```python
from build123d import *

# Parameters (mm, degrees)
SKETCH1_R                    = 4
BASE_FLANGE1_DEPTH           = 1.6002
EDGE_FLANGE1_STRIP_W         = 8.40080108
EDGE_FLANGE1_STRIP_H         = 1.6002
EDGE_FLANGE1_STRIP_CUT_DEPTH = 14
EDGE_FLANGE1_DEPTH           = 14
EDGE_FLANGE1_START           = 1.6002
EDGE_FLANGE1_PROFILE_R       = 2.5
EDGE_FLANGE1_FLAT_DEPTH      = 1.6002


# Sheet-metal steps are written as plain solids
with BuildPart() as part:
    # Sketch1 → Base-Flange1 (new body)
    with BuildSketch(Plane.XY):
        with BuildLine():
            Line((-7, -20), (-7, 0))
            ThreePointArc((-7, 0), (0, 7), (7, 0))
            Line((7, 0), (7, -20))
            Line((7, -20), (-7, -20))
        make_face()
        Circle(SKETCH1_R, mode=Mode.SUBTRACT)
    extrude(amount=-BASE_FLANGE1_DEPTH)

    # Edge-Flange1 strip (across the edge) → Edge-Flange1 strip cut (cut)
    with BuildSketch(Plane(origin=(-7, -20, 0), x_dir=(0, 1, 0), z_dir=(1, 0, 0))):
        with Locations((-3.2004, -0.8001)):
            Rectangle(EDGE_FLANGE1_STRIP_W, EDGE_FLANGE1_STRIP_H)
    extrude(amount=EDGE_FLANGE1_STRIP_CUT_DEPTH, mode=Mode.SUBTRACT)

    # Edge-Flange1 bend section (across the edge) → Edge-Flange1 (add)
    with BuildSketch(Plane(origin=(-7, -20, 0), x_dir=(0, 1, 0), z_dir=(1, 0, 0))):
        with BuildLine():
            Line((-1.6002, 1.00000054), (0, 1.00000054))
            ThreePointArc((0, 1.00000054), (0.292893377, 0.292893377), (1.00000054, 0))
            Line((1.00000054, 0), (1.00000054, -1.6002))
            ThreePointArc((1.00000054, -1.6002), (-0.838618894, -0.838618894), (-1.6002, 1.00000054))
        make_face()
    extrude(amount=EDGE_FLANGE1_DEPTH)

    # Edge-Flange1 profile (on flange) → Edge-Flange1 flat (add)
    with BuildSketch(Plane.XZ.offset(20).offset(EDGE_FLANGE1_START)):
        with BuildLine():
            ThreePointArc((7, 7), (0, 14), (-7, 7))
            Line((-7, 7), (-7, 1.00000054))
            Line((-7, 1.00000054), (7, 1.00000054))
            Line((7, 1.00000054), (7, 7))
        make_face()
        with Locations((0, 7)):
            Circle(EDGE_FLANGE1_PROFILE_R, mode=Mode.SUBTRACT)
    extrude(amount=-EDGE_FLANGE1_FLAT_DEPTH)


solid = part.part
```
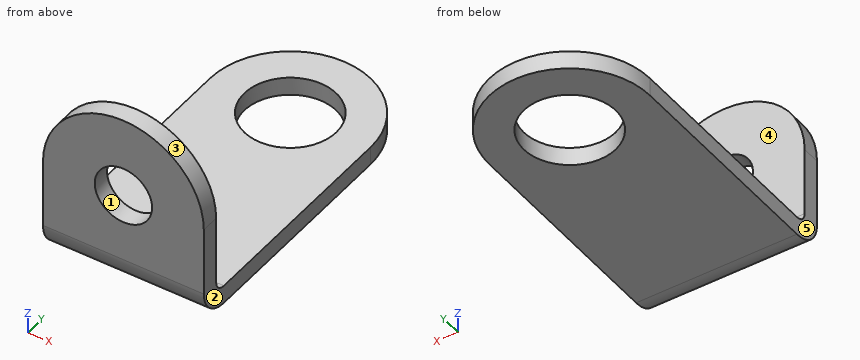
Input: part model. Units: mm. Frame: model coordinates. Face numbers are marked on the shaded views. A direction names the side the tool comes from. Coordinates: 2 decimals unless noted, no trailing zeros. Loops run counter-clockwise (first coordinate to the right, second up) from the corner with the lowest first, then second, coordinate; pieces in that order, holes last. Notation, with made-up numbers: (-12, 23) - (19, 23) arc R19 ccw to (19, 40) - close; hole circle Ø4 at (5.25, 66). An arc over 180 degrees is marked (long way). Answer in a Markdown table with one row per item.
(1) Cut plane A-A on x = 0. Output: boundary loops of the cut face in (y, z), plus the area to 3 significant figures.
Model answer:
| item | result |
|---|---|
| outline | (-21.6, 1) arc R2.6 ccw to (-19, -1.6) - (-4, -1.6) - (-4, 0) - (-19, 0) arc R1 cw to (-20, 1) - (-20, 4.5) - (-21.6, 4.5) - close; (-21.6, 9.5) - (-20, 9.5) - (-20, 14) - (-21.6, 14) - close; (4, -1.6) - (7, -1.6) - (7, 0) - (4, 0) - close |
| area | 46.1 mm² |
(2) Cut plane C-C on x = -3. Output: boundary loops of the cut face in (y, z).
Model answer:
| item | result |
|---|---|
| outline | (-21.6, 1) arc R2.6 ccw to (-19, -1.6) - (-2.65, -1.6) - (-2.65, 0) - (-19, 0) arc R1 cw to (-20, 1) - (-20, 13.32) - (-21.6, 13.32) - close; (2.65, -1.6) - (6.32, -1.6) - (6.32, 0) - (2.65, 0) - close |
(3) Mould query, pull axis Z, two halves, no side actions, for the marked faces 1, 2 and 3. Classes: pulls with the +Z half, pulls with the -Z half, needs draft (parallel to the pull), parting line crosses it, or undercut.
Model answer:
| item | result |
|---|---|
| face 1 | undercut |
| face 2 | needs draft |
| face 3 | pulls with the +Z half |
(4) Pin query (flat end, axial travel): P1, Ø7, axis at x = 2, y = -6.5, coming from the +Z side; P2, Ø4, axis at x = 3, z = 4.5, coming from the +Y side; P3, Ø3, axis at x = 0, z = 7, coming from the +Y side. Return the tip coordinate at first contact, or that it passes through.
Model answer:
| item | result |
|---|---|
| P1 | stops at z = 0 |
| P2 | stops at y = -20 |
| P3 | passes through |
(5) Material intervals for L1, parallel to Z at x = -3.75, y = -4.5; L2, parallel to Y at x = 3, z = 3.5; L3, parallel to Z at x = 0, y = -20.4, sorted ascending. Write a range as from..to.
Model answer:
| item | result |
|---|---|
| L1 | z = -1.6..0 |
| L2 | y = -21.6..-20 |
| L3 | z = -1.19..4.5, 9.5..14 |
(6) Cut plane D-D on y = -16. Output: boundary loops of the cut face in (x, z), plus the area to 3 significant figures.
Model answer:
| item | result |
|---|---|
| outline | (-7, -1.6) - (7, -1.6) - (7, 0) - (-7, 0) - close |
| area | 22.4 mm² |
(7) Cut plane B-B on z = 8.5. Output: boundary loops of the cut face in (x, y), plus the area to 3 significant figures.
Model answer:
| item | result |
|---|---|
| outline | (-6.84, -21.6) - (-2, -21.6) - (-2, -20) - (-6.84, -20) - close; (2, -21.6) - (6.84, -21.6) - (6.84, -20) - (2, -20) - close |
| area | 15.5 mm² |
(8) Set-up query: the marked faces 4 and 5. Return all of +Z, -Z, +X, -X, +Y, -Y with unobstructed straight access to the full face (end or side cutting, diameter ignored); none if empty.
Model answer:
| item | result |
|---|---|
| face 4 | +Z, +X, -X, +Y |
| face 5 | +Z, -Z, -X, +Y, -Y |
